Print and shaded views of the part. All mm, measured from the part's lowest x, y and z. A direction names the side the tool comes from. Coordinates: 2 decimals unless noted, no trailing zeros. Order: outer loops, then holes, each group sorted by start corner. A loop starts at its lowest first (then second) coordinate and runs counter-clockwise, first axis right, second up.
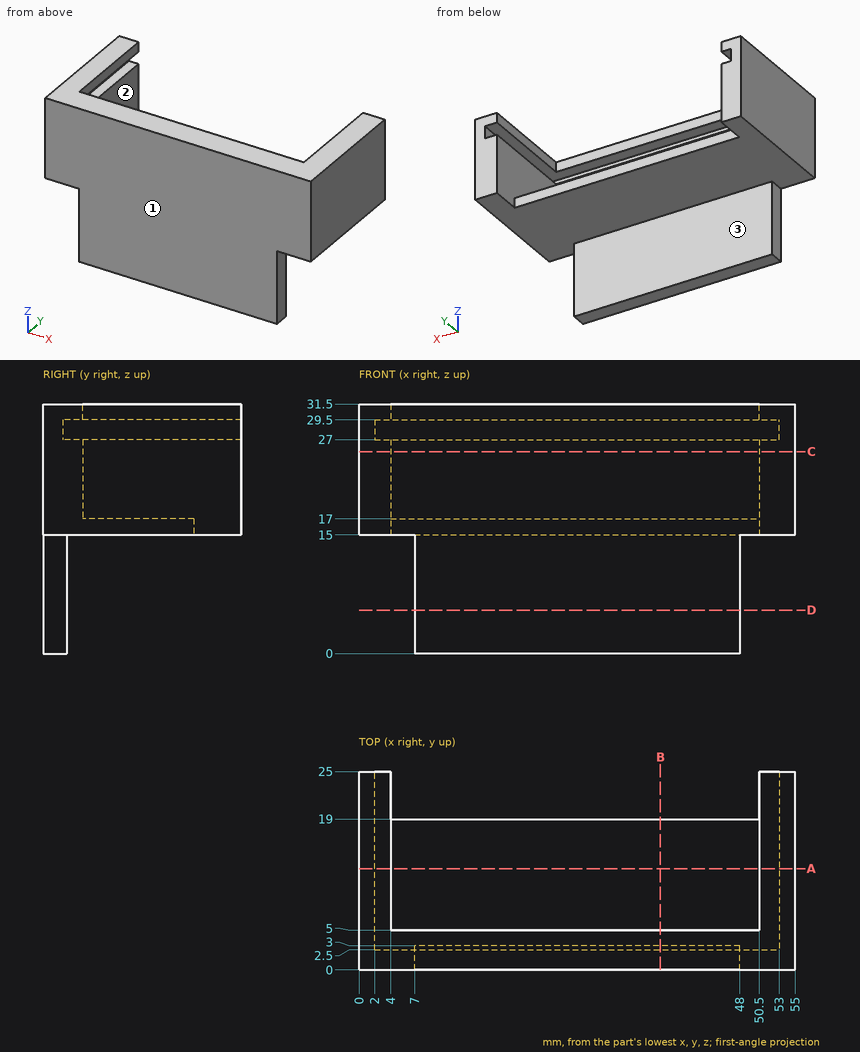
Q1. Cut at C-C, the plane z = 25.5. List the corners of the cut face in (x, y).
Established:
outline: (0, 0) - (55, 0) - (55, 25) - (50.5, 25) - (50.5, 5) - (4, 5) - (4, 25) - (0, 25) - close
Q2. Cut at D-D, the plane z = 5.5. List the corners of the cut face in (x, y).
Established:
outline: (7, 0) - (48, 0) - (48, 3) - (7, 3) - close
Q3. Cut at B-B, the plane x = 38. List the corners of the cut face in (y, z).
Established:
outline: (0, 0) - (3, 0) - (3, 15) - (19, 15) - (19, 17) - (5, 17) - (5, 27) - (2.5, 27) - (2.5, 29.5) - (5, 29.5) - (5, 31.5) - (0, 31.5) - close
Q4. Drop flat-ended pins along their axis: P1, Ø6, axis at x = 49.5, y = 6.5, coming from the +Z side; P2, Ø1.6, axis at x = 35, z = 30.5, coming from the +Y side; P3, Ø3.5, axis at y = 1, z = 4, coming from the +X side; P4, Ø12, axis at y = 11.5, z = 8, coming from the -X side. Give the stop position or say it passes through.
Established:
P1: stops at z = 31.5
P2: stops at y = 5
P3: stops at x = 48
P4: passes through
Q5. Probe line 1 (X direction, y = 5.75, z = 25.5); line 2 (Z direction, x = 25.5, y = 4); line 3 (X direction, y = 15.25, z = 28). List the from-to ranges inside material, lowest first.
Established:
line 1: x = 0 to 4, 50.5 to 55
line 2: z = 15 to 27, 29.5 to 31.5
line 3: x = 0 to 2, 53 to 55
Q6. Which spindle directions (+Z, -Z, +X, -X, +Y, -Y) get a long thin tool onto all of the face, cutting with end or side? Do the marked faces 1, 2 and 3. Say none if no direction does.
Established:
face 1: +Z, -Z, +X, -X, -Y
face 2: +Z, +Y
face 3: -Z, +X, -X, +Y
Q7. Cut at A-A, the plane y = 12.75. List the corners of the cut face in (x, z).
Established:
outline: (0, 15) - (55, 15) - (55, 31.5) - (50.5, 31.5) - (50.5, 29.5) - (53, 29.5) - (53, 27) - (50.5, 27) - (50.5, 17) - (4, 17) - (4, 27) - (2, 27) - (2, 29.5) - (4, 29.5) - (4, 31.5) - (0, 31.5) - close
